For this review, take the finished solid that the model builds, in its own axes (mm). A direction names the side the tool comes from. Give positions to 0.01 mm unless a question says otherwise; leave off trailing zeros. Loops run counter-clockwise (first coordinate to the right, second up) from the corner with the lowest first, then second, coordinate; pieces in that order, holes last.
```python
from build123d import *

# Parameters (mm, degrees)
F1_DEPTH = 63.5


with BuildPart() as f1:
    # F0 (on Front) → F1 (new body, symmetric)
    with BuildSketch(Plane.XZ):
        with BuildLine():
            add(Edge.make_bspline(
                [(-41.275, 9.525), (-40.863544, 31.082287), (9.773727, 52.372959), (48.429718, 46.904484)],
                knots=[0, 0, 0, 0, 97.18108, 97.18108, 97.18108, 97.18108], degree=3))
            Line((-41.275, 9.525), (25.213744, 9.525))
            Line((25.213744, 9.525), (25.213744, 22.997882))
            ThreePointArc((25.213744, 22.997882), (32.145966, 38.720956), (48.429718, 44.20823))
            Line((48.429718, 44.20823), (48.429718, 46.904484))
        make_face()
        Polygon((25.213744, 9.525), (-41.275, 9.525), (-41.275, -9.525), (41.275, -9.525), (41.275, 9.525), align=None)
        with BuildLine():
            Line((25.213744, 22.997882), (25.213744, 9.525))
            Line((25.213744, 9.525), (41.275, 9.525))
            Line((41.275, 9.525), (41.275, 22.997882))
            ThreePointArc((41.275, 22.997882), (43.564075, 27.325707), (48.429718, 27.869256))
            Line((48.429718, 27.869256), (48.429718, 44.20823))
            ThreePointArc((48.429718, 44.20823), (32.145966, 38.720956), (25.213744, 22.997882))
        make_face()
        Polygon((72.02662, 46.904484), (48.429718, 46.904484), (48.429718, 44.20823), (48.429718, 27.869256), (48.429718, 18.329484), (72.02662, 18.329484), align=None)
    extrude(amount=F1_DEPTH, both=True)


solid = f1.part
```
Item 1: Take a section at A-A on z = 4.5. Give the boundary of the cut face in (x, y) (3 decimals), and give its area (3 significant figures).
Answer:
outline: (-41.275, -63.5) - (41.275, -63.5) - (41.275, 63.5) - (-41.275, 63.5) - close
area: 10,500 mm2
Item 2: Clearance check with flat-ended pins moving along their axes: pin 1 Ø10 at (y, z) = (28, 12.5) entering from +X (3 decimals); pin 2 Ø6 at (x, y) = (20.5, -45.5) entering from +Z; pin 3 Ø5 at (y, z) = (22.5, 24.5) entering from -X. State where each tip first meets the part, or that it passes through.
Answer:
pin 1: stops at x = 41.275
pin 2: stops at z = 47.1
pin 3: stops at x = -35.69
Item 3: For L1, parallel to Z at x = 66.5, y = -32; L2, parallel to X at y = 24.5, z = 1 (3 decimals); L3, parallel to Z at x = 35, y = 46 (3 decimals), list the stretches that pass through material, from the lowest coordinate up.
Answer:
L1: z = 18.33 to 46.9
L2: x = -41.275 to 41.275
L3: z = -9.525 to 47.772
Item 4: The part is to be moulded in two halves that separate along X. For faces 4 (the flat face through (-41.275, -1, 0)), 5 (the cylindrical face through (43.51, -0.89, 27.29)), 6 (the flat face through (72.027, -1, 32)), say which applies: released by +X, released by -X, zero draft, split by the parting line, or undercut.
Answer:
face 4: released by -X
face 5: undercut
face 6: released by +X
Item 5: Tool access review of faces 1 (the flat face through (48.43, -1, 23)), 2 (the flat face through (60, -1, 18.329)), 3 (the flat face through (60, -1, 46.904)): name each direction out of +Z, -Z, +X, -X, +Y, -Y from which nothing blocks a thin tool from reaching the whole face with its end or side.
Answer:
face 1: -Z, +Y, -Y
face 2: -Z, +X, +Y, -Y
face 3: +Z, +X, +Y, -Y
